Work out the finished part from the listing and answer in its coordinate system (mm). Face numbers are marked on the shaded views. A direction names the side the tool comes from. Round coordinates to 2 decimals unless told otherwise and drop trailing zeros. Order: outer loops, then holes, each group sorted by start corner. A loop starts at its lowest first (then second) coordinate and runs counter-clockwise, first axis right, second up. Notation, with made-up numbers: M 54.5,85.5 L 69.5,85.5 A10 cw 69.5,98.5 Z; hole C 57.25,34.25 d10. An arc over 180 degrees is marked long. Return JSON: item names as keys, results as strings.
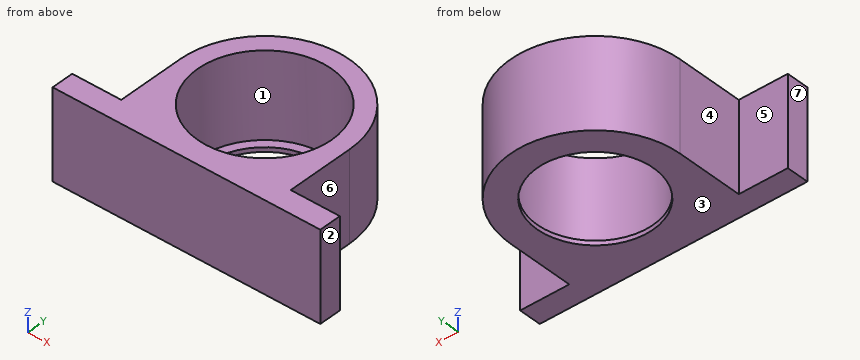
from build123d import *

# Parameters (mm, degrees)
SKETCH_R     = 15
PAD_DEPTH    = 20
SKETCH001_R  = 13
PAD001_DEPTH = 1


with BuildPart() as part:
    # Sketch → Pad (new body)
    with BuildSketch(Plane.XY):
        with BuildLine():
            Line((30, 5), (30, 0))
            Line((30, 0), (-30, 0))
            Line((-30, 0), (-30, 5))
            Line((-30, 5), (-19, 5))
            Line((-19, 20), (-19, 5))
            ThreePointArc((19, 20), (0, 39), (-19, 20))
            Line((19, 20), (19, 5))
            Line((19, 5), (30, 5))
        make_face()
        with Locations((0, 20)):
            Circle(SKETCH_R, mode=Mode.SUBTRACT)
    extrude(amount=PAD_DEPTH)

    # Sketch001 (on Face10 of Pad) → Pad001 (join)
    with BuildSketch(Plane(origin=(0, 0, 0), x_dir=(1, 0, 0), z_dir=(0, 0, -1))):
        with BuildLine():
            ThreePointArc((-19, -20), (0, -39), (19, -20))
            Line((19, -5), (19, -20))
            Line((30, -5), (19, -5))
            Line((30, 0), (30, -5))
            Line((-30, 0), (30, 0))
            Line((-30, -5), (-30, 0))
            Line((-19, -5), (-30, -5))
            Line((-19, -20), (-19, -5))
        make_face()
        with Locations((0, -20)):
            Circle(SKETCH001_R, mode=Mode.SUBTRACT)
    extrude(amount=-PAD001_DEPTH)


solid = part.part
Item 1: Find section A-A (z = 16). Determine the outline of the cut face in (x, y).
Output:
{"outline": "M -30,0 L 30,0 L 30,5 L 19,5 L 19,20 A19 ccw -19,20 L -19,5 L -30,5 Z; hole C 0,20 d30"}
Item 2: Find section C-C (y = 25.5). Determine the outline of the cut face in (x, z), plus the area to 3 significant figures.
Output:
{"outline": "M -18.19,0 L -11.78,0 L -11.78,1 L -13.96,1 L -13.96,20 L -18.19,20 Z; M 11.78,0 L 18.19,0 L 18.19,20 L 13.96,20 L 13.96,1 L 11.78,1 Z", "area": "174 mm^2"}
Item 3: Each of these flat-tipped pins is pushed along its axis until it touches: pin 1 (5 mm diameter, centred on x = 2, z = 16, fed in from +Y); pin 2 (15 mm diameter, centred on x = 2, y = 19.5, fed in from +Z); pin 3 (2 mm diameter, centred on y = 7, z = 12, fed in from +X); pin 4 (3.5 mm diameter, centred on x = 25.5, z = 14, fed in from +Y). Where does it stop, or does it pass through?
Output:
{"pin 1": "stops at y = 39", "pin 2": "passes through", "pin 3": "stops at x = 19", "pin 4": "stops at y = 5"}
Item 4: Which of the six approach directions +Z, -Z, +X, -X, +Y, -Y give full straight-line access (tool end or side, diameter ignored) to the marked faces 5, 6 and 7?
Output:
{"face 5": "+Z, -Z, -X, +Y", "face 6": "+Z, -Z, +X, +Y", "face 7": "+Z, -Z, -X, +Y, -Y"}
Item 5: Consider line 1 along Y through (x, z) = (0, 12.25); line 2 along X through (y, z) = (20, 0.6); line 3 along Y through (x, z) = (0, 0.8). Determine where each line is inside the solid, lowest interval first. Write a range as [from, to].
Output:
{"line 1": "y = [0, 5], [35, 39]", "line 2": "x = [-19, -13], [13, 19]", "line 3": "y = [0, 7], [33, 39]"}
Item 6: Find section D-D (x = 25). Determine the outline of the cut face in (y, z).
Output:
{"outline": "M 0,0 L 5,0 L 5,20 L 0,20 Z"}
Item 7: Find section B-B (x = 0). Determine the outline of the cut face in (y, z).
Output:
{"outline": "M 0,0 L 7,0 L 7,1 L 5,1 L 5,20 L 0,20 Z; M 33,0 L 39,0 L 39,20 L 35,20 L 35,1 L 33,1 Z"}
Item 8: The mould has two halves that part along X. Classify the marked faces 1, 2, 3 and 4: pulls with the +X half, pulls with the -X half, needs draft (parallel to the pull), parting line crosses it, or undercut.
Output:
{"face 1": "undercut", "face 2": "pulls with the +X half", "face 3": "needs draft", "face 4": "pulls with the -X half"}
